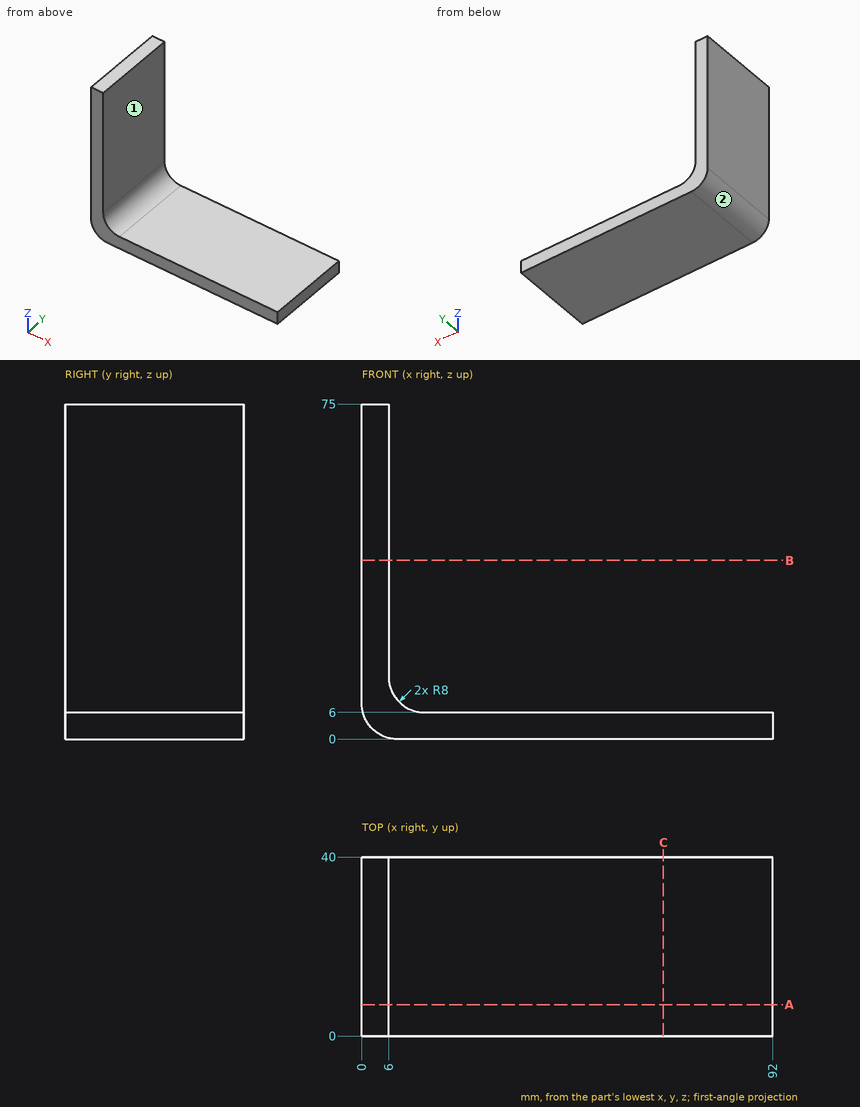
Geometry check sheet. Reference: drawing and pictorial views, mm from the part's lowest x, y, z. A direction names the side the tool comes from. Coordinates: 2 decimals unless noted, no trailing zeros. Order: outer loops, then holes, each group sorted by start corner. A loop starts at its lowest first (then second) coordinate and runs counter-clockwise, first axis right, second up.
Item 1: Scan lines: line 1 along Z through (x, y) = (14, 22); line 2 along X through (y, z) = (25.5, 11). Record each from-to range of solid material in increasing order.
Item 2: Depth check by flat-ended pin: pin 1 (8 mm diameter, centred on x = 66, y = 22, fed in from -Z); pin 2 (12 mm diameter, centred on x = 42.5, y = 27.5, fed in from +Z); pin 3 (5 mm diameter, centred on y = 17.5, z = 49.5, fed in from +X). Enter the tip coordinate at first touch or a pass-through.
Item 3: Section check C-C (x = 67.5). Enter the section's corners in (y, z).
Item 4: Section check B-B (z = 40). Enter the section's corners in (x, y), plus the area to 3 significant figures.
Item 5: Section check A-A (y = 7). Enter the section's corners in (x, z).
Item 6: Tool access check on the marked faces 1 and 2. Record the directions out of +Z, -Z, +X, -X, +Y, -Y that give a thin tool (end or side, any length) a straight path to the whole face; none if there is none.
Check sheet entries:
1. line 1: z = 0 to 6
1. line 2: x = 0 to 6.58
2. pin 1: stops at z = 0
2. pin 2: stops at z = 6
2. pin 3: stops at x = 6
3. outline: (0, 0) - (40, 0) - (40, 6) - (0, 6) - close
4. outline: (0, 0) - (6, 0) - (6, 40) - (0, 40) - close
4. area: 240 mm2
5. outline: (0, 8) arc R8 ccw to (8, 0) - (92, 0) - (92, 6) - (14, 6) arc R8 cw to (6, 14) - (6, 75) - (0, 75) - close
6. face 1: +Z, +X, +Y, -Y
6. face 2: -Z, -X, +Y, -Y
